from build123d import *

# Parameters (mm, degrees)
SKETCH3_W           = 63.25
SKETCH3_H           = 63.25
SKETCH3_W_2         = 10
SKETCH3_H_2         = 10
BOSS_EXTRUDE3_DEPTH = 2


with BuildPart() as part:
    # Sketch3 → Boss-Extrude3 (new body)
    with BuildSketch(Plane(origin=(0, 0, 0), x_dir=(1, 0, 0), z_dir=(0, 1, 0))):
        with Locations((0.125, 0.125)):
            Rectangle(SKETCH3_W, SKETCH3_H)
        with Locations((-12.245, 24.875)):
            Rectangle(SKETCH3_W_2, SKETCH3_H_2, mode=Mode.SUBTRACT)
        with Locations((-24.625, 24.875)):
            Rectangle(SKETCH3_W_2, SKETCH3_H_2, mode=Mode.SUBTRACT)
        with Locations((0.135, 24.875)):
            Rectangle(SKETCH3_W_2, SKETCH3_H_2, mode=Mode.SUBTRACT)
        with Locations((12.515, 24.875)):
            Rectangle(SKETCH3_W_2, SKETCH3_H_2, mode=Mode.SUBTRACT)
        with Locations((24.895, 24.875)):
            Rectangle(SKETCH3_W_2, SKETCH3_H_2, mode=Mode.SUBTRACT)
        with Locations((-12.245, 12.495)):
            Rectangle(SKETCH3_W_2, SKETCH3_H_2, mode=Mode.SUBTRACT)
        with Locations((0.135, 12.495)):
            Rectangle(SKETCH3_W_2, SKETCH3_H_2, mode=Mode.SUBTRACT)
        with Locations((12.515, 12.495)):
            Rectangle(SKETCH3_W_2, SKETCH3_H_2, mode=Mode.SUBTRACT)
        with Locations((24.895, 12.495)):
            Rectangle(SKETCH3_W_2, SKETCH3_H_2, mode=Mode.SUBTRACT)
        with Locations((-12.245, 0.115)):
            Rectangle(SKETCH3_W_2, SKETCH3_H_2, mode=Mode.SUBTRACT)
        with Locations((0.135, 0.115)):
            Rectangle(SKETCH3_W_2, SKETCH3_H_2, mode=Mode.SUBTRACT)
        with Locations((12.515, 0.115)):
            Rectangle(SKETCH3_W_2, SKETCH3_H_2, mode=Mode.SUBTRACT)
        with Locations((24.895, 0.115)):
            Rectangle(SKETCH3_W_2, SKETCH3_H_2, mode=Mode.SUBTRACT)
        with Locations((-12.245, -12.265)):
            Rectangle(SKETCH3_W_2, SKETCH3_H_2, mode=Mode.SUBTRACT)
        with Locations((0.135, -12.265)):
            Rectangle(SKETCH3_W_2, SKETCH3_H_2, mode=Mode.SUBTRACT)
        with Locations((12.515, -12.265)):
            Rectangle(SKETCH3_W_2, SKETCH3_H_2, mode=Mode.SUBTRACT)
        with Locations((24.895, -12.265)):
            Rectangle(SKETCH3_W_2, SKETCH3_H_2, mode=Mode.SUBTRACT)
        with Locations((-12.245, -24.645)):
            Rectangle(SKETCH3_W_2, SKETCH3_H_2, mode=Mode.SUBTRACT)
        with Locations((0.135, -24.645)):
            Rectangle(SKETCH3_W_2, SKETCH3_H_2, mode=Mode.SUBTRACT)
        with Locations((12.515, -24.645)):
            Rectangle(SKETCH3_W_2, SKETCH3_H_2, mode=Mode.SUBTRACT)
        with Locations((24.895, -24.645)):
            Rectangle(SKETCH3_W_2, SKETCH3_H_2, mode=Mode.SUBTRACT)
        with Locations((-24.625, 12.495)):
            Rectangle(SKETCH3_W_2, SKETCH3_H_2, mode=Mode.SUBTRACT)
        with Locations((-24.625, 0.115)):
            Rectangle(SKETCH3_W_2, SKETCH3_H_2, mode=Mode.SUBTRACT)
        with Locations((-24.625, -12.265)):
            Rectangle(SKETCH3_W_2, SKETCH3_H_2, mode=Mode.SUBTRACT)
        with Locations((-24.625, -24.645)):
            Rectangle(SKETCH3_W_2, SKETCH3_H_2, mode=Mode.SUBTRACT)
    extrude(amount=BOSS_EXTRUDE3_DEPTH)


solid = part.part
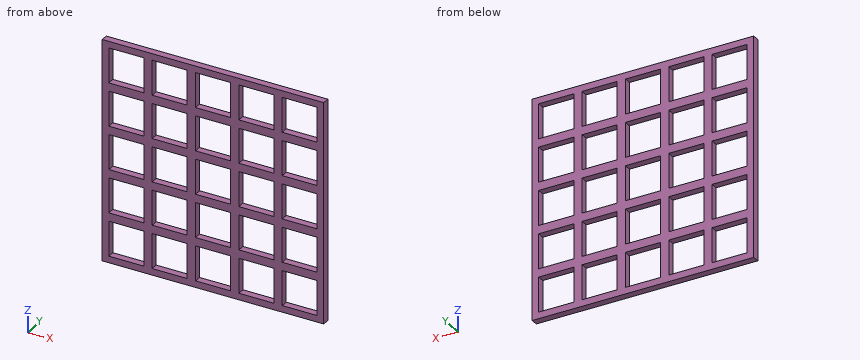
Work out the finished part from the listing and answer in its coordinate system (mm). Give positions to 0.01 mm unless a question says otherwise; leave off trailing zeros. Loops run counter-clockwise (first coordinate to the right, second up) from the corner with the lowest first, then second, coordinate; pieces in that order, holes last. Notation, with made-up numbers: (7, 61.25) -> (35, 61.25) arc R11 cw to (35, 66.25) -> close; hole circle Ø3 at (-37.75, 39.25). An arc over 180 degrees is marked (long way). Use a Markdown table: item, result. Add a question column.
1. Section A-A on z = -23.5 is taken. Determine the outline of the cut face in (x, y) (3 decimals).
2. Find the intervals of material crossed by probe 1 along Z at (x, y) = (20, 0.85) (3 decimals); probe 2 along X at (y, z) = (1.05, -27) (3 decimals), in increasing order.
3. Section B-B on x = 22.5 is taken. Determine the outline of the cut face in (y, z) (3 decimals).
4. Section C-C on y = 1.4 is taken. State how many separate pieces and enclosed holes the cut face has, and give its area (3 significant figures).
Results below:
| question | item | result |
|---|---|---|
| 1 | outline | (-31.5, 0) -> (-29.625, 0) -> (-29.625, 2) -> (-31.5, 2) -> close; (-19.625, 0) -> (-17.245, 0) -> (-17.245, 2) -> (-19.625, 2) -> close; (-7.245, 0) -> (-4.865, 0) -> (-4.865, 2) -> (-7.245, 2) -> close; (5.135, 0) -> (7.515, 0) -> (7.515, 2) -> (5.135, 2) -> close; (17.515, 0) -> (19.895, 0) -> (19.895, 2) -> (17.515, 2) -> close; (29.895, 0) -> (31.75, 0) -> (31.75, 2) -> (29.895, 2) -> close |
| 2 | probe 1 | z = -31.75 to -29.875, -19.875 to -17.495, -7.495 to -5.115, 4.885 to 7.265, 17.265 to 19.645, 29.645 to 31.5 |
| 2 | probe 2 | x = -31.5 to -29.625, -19.625 to -17.245, -7.245 to -4.865, 5.135 to 7.515, 17.515 to 19.895, 29.895 to 31.75 |
| 3 | outline | (0, -31.75) -> (2, -31.75) -> (2, -29.875) -> (0, -29.875) -> close; (0, -19.875) -> (2, -19.875) -> (2, -17.495) -> (0, -17.495) -> close; (0, -7.495) -> (2, -7.495) -> (2, -5.115) -> (0, -5.115) -> close; (0, 4.885) -> (2, 4.885) -> (2, 7.265) -> (0, 7.265) -> close; (0, 17.265) -> (2, 17.265) -> (2, 19.645) -> (0, 19.645) -> close; (0, 29.645) -> (2, 29.645) -> (2, 31.5) -> (0, 31.5) -> close |
| 4 | separate pieces | 1 |
| 4 | enclosed holes | 25 |
| 4 | area | 1,500 mm^2 |
